For this review, use the dimensioned drawing (mm, ordinates from the lowest corner) and the shaded views. A direction names the side the tool comes from. Coordinates: 2 decimals unless noted, no trailing zeros. Write each loop counter-clockwise with the first axis right and the second up, starting at its lowest first coordinate (ties: lowest second). Pieces come first, ordered by that corner, then holes. Notation, with made-up numbers: (81, 39) -> (88, 39) arc R9 ccw to (88, 46) -> close; hole circle Ø1 at (-2, 46). An arc over 180 degrees is marked (long way). Put each result on its own line as item: value. Start each with the question number.
Item 1: Consider section C-C on z = 11.25. Give the boundary of the cut face in (x, y).
Item 2: For the marked faces 1, 2 and 3, list the 3-axis set-ups (+Z, -Z, +X, -X, +Y, -Y) from which the entire face can be reached by the end or side of a thin tool; tool diameter is ignored.
Item 3: Consider section B-B on y = 2.2. Give the boundary of the cut face in (x, z).
Item 4: To check wall thickness, follow L1, parallel to X at y = 3.7, z = 27.5; L2, parallel to Z at x = 9.25, y = 1.3; L3, parallel to X at y = 2.1, z = 16. State the ranges of each line that lie inside material, in increasing order.
Item 5: Consider section D-D on x = 27.5. Give the boundary of the cut face in (y, z).
Item 6: Consider section A-A on x = 18.5. Give the boundary of the cut face in (y, z), and give its area (3 significant figures).
Item 7: Insertion check: P1, Ø1.2, axis at x = 16, y = 2, coming from the +Z side; P2, Ø1.5, axis at y = 3, z = 15.5, coming from the +X side; P3, Ø2, axis at x = 19, y = 2.5, coming from the +Z side. Each pin has a flat end and moves straight along its axis. Give the tip position at first contact, or say it passes through.
Item 8: The part is to be moulded in two halves that separate along X. For the marked faces 4, 5 and 6, say which applies: +X half, -X half, draft (parallel to the pull), parting line (faces both ways), or undercut.
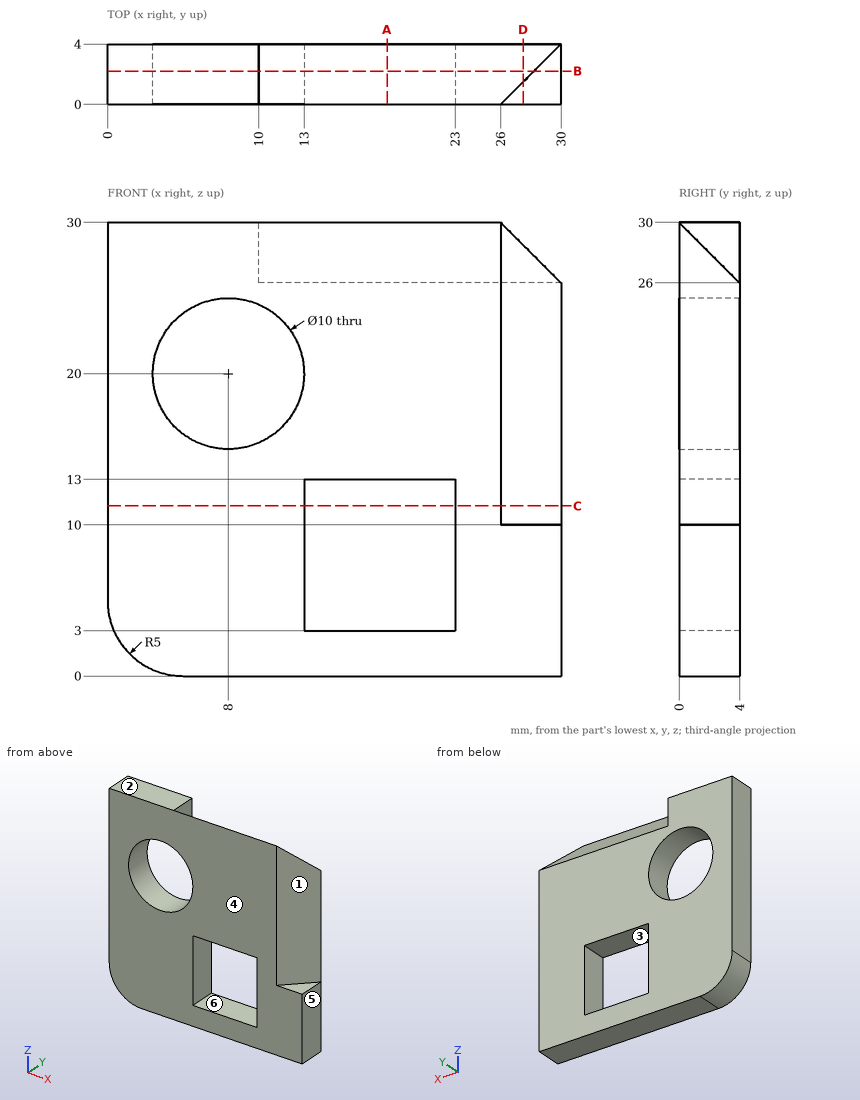
Return value:
1. outline: (0, 0) -> (13, 0) -> (13, 4) -> (0, 4) -> close; (23, 0) -> (26, 0) -> (30, 4) -> (23, 4) -> close
2. face 1: +Z, +X, -Y
2. face 2: +Z, +X, -X, +Y, -Y
2. face 3: +Y, -Y
3. outline: (0, 5) arc R5 ccw to (5, 0) -> (30, 0) -> (30, 10) -> (28.2, 10) -> (28.2, 27.8) -> (10, 27.8) -> (10, 30) -> (0, 30) -> close; hole circle Ø10 at (8, 20); hole (13, 3) -> (23, 3) -> (23, 13) -> (13, 13) -> close
4. L1: 0 to 10
4. L2: 0 to 15.16, 24.84 to 30
4. L3: 0 to 5, 11 to 28.1
5. outline: (0, 0) -> (4, 0) -> (4, 26) -> (1.5, 28.5) -> (1.5, 10) -> (0, 10) -> close
6. outline: (0, 0) -> (4, 0) -> (4, 3) -> (0, 3) -> close; (0, 13) -> (4, 13) -> (4, 26) -> (0, 30) -> close
6. area: 72.0 mm^2
7. P1: z = 28.6
7. P2: x = 29.75
7. P3: z = 28.5
8. face 4: draft
8. face 5: +X half
8. face 6: undercut
